The model under review builds one solid part; all positions refer to its coordinate system, in mm. Face numbers are marked on the shaded views. A direction names the side the tool comes from. Round coordinates to 2 decimals unless told otherwise and drop trailing zeros. Order: outer loops, then holes, each group sorted by start corner. A loop starts at its lowest first (then second) coordinate and runs counter-clockwise, first axis right, second up. Notation, with made-up numbers: M 63,2 L 117,2 A26 ccw 117,17 Z; hole C 89.25,81.25 d11. An arc over 180 degrees is marked long. Use a Markdown table: item, result. Add a question column.
1. Consider section D-D on z = 1. State the section outline as (x, y) points.
2. To check wall thickness, follow probe 1 along X at (y, z) = (4.9, 1.25); probe 2 along Y at (x, z) = (-1.65, 4.25); probe 3 along Y at (x, z) = (-0.7, 3.25). State the ranges of each line that lie inside material, in increasing order.
3. Consider section B-B on y = 5.4. State the section outline as (x, z) points, then the cut area to 3 significant figures.
4. Consider section C-C on y = 2.95. State the section outline as (x, z) points, then the cut area to 3 significant figures.
5. The part is to be moulded in two halves that separate along Z. For the marked faces 1, 2, 3 and 4, say which applies: +Z half, -Z half, draft (parallel to the pull), parting line (faces both ways), or undercut.
6. For the marked faces 5 and 6, list the 3-axis set-ups (+Z, -Z, +X, -X, +Y, -Y) from which the entire face can be reached by the end or side of a thin tool; tool diameter is ignored.
7. Consider section A-A on x = -1. State the section outline as (y, z) points.
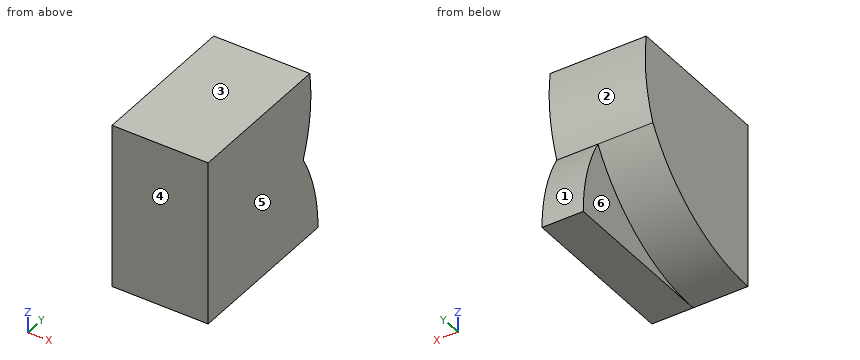
from build123d import *

# Parameters (mm, degrees)
BOSS_EXTRUDE1_DEPTH = 1.5
BOSS_EXTRUDE2_DEPTH = 3.5
BOSS_EXTRUDE3_DEPTH = 3.5
BOSS_EXTRUDE4_DEPTH = 3.5


with BuildPart() as part:
    # Sketch1 → Boss-Extrude1 (new body)
    with BuildSketch(Plane(origin=(0, 0, 0), x_dir=(0, 0, -1), z_dir=(1, 0, 0))):
        with BuildLine():
            Line((-3, 5.196152423), (-3, 0))
            Line((-3, 0), (0, 0))
            Line((0, 0), (0, 6))
            ThreePointArc((0, 6), (-1.552914271, 5.795554958), (-3, 5.196152423))
        make_face()
    extrude(amount=-BOSS_EXTRUDE1_DEPTH)

    # Sketch2 → Boss-Extrude2 (add)
    with BuildSketch(Plane(origin=(0, 0, 0), x_dir=(0, 0, -1), z_dir=(1, 0, 0))):
        with BuildLine():
            Line((-3, 0), (-6.023586903, 0))
            ThreePointArc((-6.023586903, 0), (-5.20953131, 3.004082594), (-3, 5.196152423))
            Line((-3, 5.196152423), (-3, 0))
        make_face()
    extrude(amount=-BOSS_EXTRUDE2_DEPTH)

    # Sketch3 → Boss-Extrude3 (add)
    with BuildSketch(Plane.ZY.offset(3.5)):
        with BuildLine():
            ThreePointArc((3, 5.196152423), (0.803847577, 3), (0, 0))
            Line((0, 0), (3, 0))
            Line((3, 0), (3, 5.196152423))
        make_face()
    extrude(amount=-BOSS_EXTRUDE3_DEPTH)

    # Sketch4 → Boss-Extrude4 (add)
    with BuildSketch(Plane.ZY.offset(3.5)):
        with BuildLine():
            Line((6.023586903, 0), (6.023586903, 5.554981031))
            ThreePointArc((6.023586903, 5.554981031), (4.488653077, 5.570553782), (3, 5.196152423))
            Line((3, 5.196152423), (3, 0))
            Line((3, 0), (6.023586903, 0))
        make_face()
    extrude(amount=-BOSS_EXTRUDE4_DEPTH)


solid = part.part
Answer block:
| question | item | result |
|---|---|---|
| 1 | outline | M -3.5,0 L 0,0 L 0,5.92 L -1.5,5.92 L -1.5,3.32 L -3.5,3.32 Z |
| 2 | probe 1 | -1.5 to 0 |
| 2 | probe 2 | 0 to 5.54 |
| 2 | probe 3 | 0 to 5.29 |
| 3 | outline | M -3.5,3.61 L 0,3.61 L 0,6.02 L -3.5,6.02 Z; M -1.5,0 L 0,0 L 0,2.62 L -1.5,2.62 Z |
| 3 | area | 12.4 mm^2 |
| 4 | outline | M -3.5,0.78 L -1.5,0.78 L -1.5,0 L 0,0 L 0,6.02 L -3.5,6.02 Z |
| 4 | area | 19.5 mm^2 |
| 5 | face 1 | undercut |
| 5 | face 2 | undercut |
| 5 | face 3 | +Z half |
| 5 | face 4 | draft |
| 6 | face 5 | +Z, -Z, +X, +Y, -Y |
| 6 | face 6 | -Z, -X, +Y |
| 7 | outline | M 0,0 L 6,0 A6 ccw 5.2,3 A6 ccw 5.55,6.02 L 0,6.02 Z |
